Geometry: final body of the model. Coordinates: model frame, mm. A direction names the side the tool comes from. Give positions to 0.01 mm unless a question says otherwise; leave off trailing zeros. Order: outer loops, then holes, each group sorted by start corner. A loop starts at its lowest first (then second) coordinate and runs counter-clockwise, first axis right, second up. Notation, with made-up numbers: (57.25, 58.5) -> (115.25, 58.5) arc R23 cw to (115.25, 91.5) -> close; hole circle Ø4 at (-7.5, 74). An arc over 180 degrees is marked (long way). One line per question, with ' | ' between items.
from build123d import *

# Parameters (mm, degrees)
SKETCH1_R           = 13.97
BOSS_EXTRUDE2_DEPTH = 6.0000007
CUT_EXTRUDE1_DEPTH  = 3.81
SKETCH3_R           = 31.75
CUT_EXTRUDE2_DEPTH  = 0.3
SKETCH5_R           = 25.019
SKETCH5_R_2         = 13.97
BOSS_EXTRUDE3_DEPTH = 6.35
CUT_EXTRUDE3_START  = -0.3
SKETCH6_R           = 50.8
SKETCH6_R_2         = 31.75
CUT_EXTRUDE3_DEPTH  = 0.3


with BuildPart() as part:
    # Sketch1 → Boss-Extrude2 (new body)
    with BuildSketch(Plane(origin=(0, 0, 0), x_dir=(1, 0, 0), z_dir=(0, 1, 0))):
        with BuildLine():
            Line((35.405449863, 6.5405), (38.565312338, 6.5405))
            ThreePointArc((38.565312338, 6.5405), (27.795594479, 27.522107178), (6.9215, 38.498757042))
            Line((6.9215, 38.498757042), (6.9215, 35.332942957))
            ThreePointArc((6.9215, 35.332942957), (0.19391896, 36.003977776), (-6.5405, 35.405449863))
            Line((-6.5405, 35.405449863), (-6.5405, 38.565312338))
            ThreePointArc((-6.5405, 38.565312338), (-27.522107178, 27.795594479), (-38.498757042, 6.9215))
            Line((-38.498757042, 6.9215), (-35.332942957, 6.9215))
            ThreePointArc((-35.332942957, 6.9215), (-36.003977776, 0.19391896), (-35.405449863, -6.5405))
            Line((-35.405449863, -6.5405), (-38.565312338, -6.5405))
            ThreePointArc((-38.565312338, -6.5405), (-27.795594479, -27.522107178), (-6.9215, -38.498757042))
            Line((-6.9215, -38.498757042), (-6.9215, -35.332942957))
            ThreePointArc((-6.9215, -35.332942957), (-0.19391896, -36.003977776), (6.5405, -35.405449863))
            Line((6.5405, -35.405449863), (6.5405, -38.565312338))
            ThreePointArc((6.5405, -38.565312338), (27.522107178, -27.795594479), (38.498757042, -6.9215))
            Line((38.498757042, -6.9215), (35.332942957, -6.9215))
            ThreePointArc((35.332942957, -6.9215), (36.003977776, -0.19391896), (35.405449863, 6.5405))
        make_face()
        with Locations(Location((0, 0, 0), (0, 0, 270))):
            Circle(SKETCH1_R, mode=Mode.SUBTRACT)
    extrude(amount=BOSS_EXTRUDE2_DEPTH)

    # Sketch2 → Cut-Extrude1 (cut)
    with BuildSketch(Plane.XZ):
        with BuildLine():
            Line((17.377665752, -10.033), (-0.286554615, -40.628327152))
            ThreePointArc((-0.286554615, -40.628327152), (-2.416432138, -40.557415308), (-4.539661745, -40.374924792))
            Line((-4.539661745, -40.374924792), (8.196212586, -18.315743371))
            ThreePointArc((8.196212586, -18.315743371), (-13.440862054, 14.899247741), (17.377665752, -10.033))
        make_face()
    extrude(amount=-CUT_EXTRUDE1_DEPTH, mode=Mode.SUBTRACT)

    # Sketch3 → Cut-Extrude2 (cut)
    with BuildSketch(Plane.XZ):
        Circle(SKETCH3_R)
    extrude(amount=-CUT_EXTRUDE2_DEPTH, mode=Mode.SUBTRACT)

    # Sketch5 → Boss-Extrude3 (add)
    with BuildSketch(Plane(origin=(0, 6.0000007, 0), x_dir=(1, 0, 0), z_dir=(0, 1, 0))):
        with Locations(Location((0, 0, 0), (0, 0, 270))):
            Circle(SKETCH5_R)
        with Locations(Location((0, 0, 0), (0, 0, 270))):
            Circle(SKETCH5_R_2, mode=Mode.SUBTRACT)
    extrude(amount=BOSS_EXTRUDE3_DEPTH)

    # Sketch6 → Cut-Extrude3 (cut)
    with BuildSketch(Plane(origin=(0, 6.0000007, 0), x_dir=(1, 0, 0), z_dir=(0, 1, 0)).offset(CUT_EXTRUDE3_START)):
        Circle(SKETCH6_R)
        with Locations(Location((0, 0, 0), (0, 0, 270))):
            Circle(SKETCH6_R_2, mode=Mode.SUBTRACT)
    extrude(amount=CUT_EXTRUDE3_DEPTH, mode=Mode.SUBTRACT)


solid = part.part
1) Pull-direction query (X, two-part tool) for faces 4 (the flat face through (-6.922, 3, 37)), 5 (the cylindrical face through (27.283, 2.81, 28.031)), 6 (the flat face through (-32, 5.7, -6)); classes: +X half, -X half, draft (parallel to the pull), parting line (faces both ways), or undercut.
Check result:
face 4: undercut | face 5: +X half | face 6: draft
2) Section B-B on x = -4. Return loops of the section in (y, z).
Check result:
outline: (0, -35.78) -> (5.7, -35.78) -> (5.7, -31.5) -> (6, -31.5) -> (6, -24.7) -> (12.35, -24.7) -> (12.35, -13.39) -> (3.81, -13.39) -> (3.81, -19.66) -> (0.3, -19.66) -> (0.3, -31.5) -> (0, -31.5) -> close; (0, 31.5) -> (0.3, 31.5) -> (0.3, 19.66) -> (3.81, 19.66) -> (3.81, 13.39) -> (12.35, 13.39) -> (12.35, 24.7) -> (6, 24.7) -> (6, 31.5) -> (5.7, 31.5) -> (5.7, 35.78) -> (0, 35.78) -> close
3) Material intervals for probe 1 along X at (y, z) = (9, 0); probe 2 along Y at (x, z) = (-14.5, 17); probe 3 along X at (y, z) = (1.75, 0), sorted ascending. Write a range as from..to.
Check result:
probe 1: x = -25.02..-13.97, 13.97..25.02 | probe 2: y = 0.3..12.35 | probe 3: x = -36..-20.07, 20.07..36
4) Section A-A on z = 0. Return loops of the section in (x, y).
Check result:
outline: (-36, 0) -> (-31.75, 0) -> (-31.75, 0.3) -> (-20.07, 0.3) -> (-20.07, 3.81) -> (-13.97, 3.81) -> (-13.97, 12.35) -> (-25.02, 12.35) -> (-25.02, 6) -> (-31.75, 6) -> (-31.75, 5.7) -> (-36, 5.7) -> close; (13.97, 3.81) -> (20.07, 3.81) -> (20.07, 0.3) -> (31.75, 0.3) -> (31.75, 0) -> (36, 0) -> (36, 5.7) -> (31.75, 5.7) -> (31.75, 6) -> (25.02, 6) -> (25.02, 12.35) -> (13.97, 12.35) -> close
5) Section D-D on y = 10. Return loops of the section in (x, z).
Check result:
outline: circle Ø50.04 at (0, 0); hole circle Ø27.94 at (0, 0)
6) Set-up query: faces 1 (the flat face through (-6.54, 3, -37)), 2 (the flat face through (23.4, 6, -9.6)), 3 (the flat face through (10.009, 1.878, -22.796)). Return all of +Z, -Z, +X, -X, +Y, -Y with unobstructed straight access to the full face (end or side cutting, diameter ignored); none if empty.
Check result:
face 1: -Z, +Y, -Y | face 2: +Y | face 3: -Y
7) Contact query for flat-ended pins moving along their axis: pin 1 Ø2.5 at (y, z) = (1.5, -36.5) entering from +X; pin 2 Ø0.9 at (y, z) = (2.5, 36) entering from +X; pin 3 Ø12 at (x, z) = (-1, -8) entering from -Y. Output: stop coordinate, or through.
Check result:
pin 1: stops at x = 16.96 | pin 2: stops at x = 16.32 | pin 3: stops at y = 3.81
8) Section C-C on x = 21. Return loops of the section in (y, z), plus the area to 3 significant figures.
Check result:
outline: (0, -33) -> (5.7, -33) -> (5.7, -23.81) -> (6, -23.81) -> (6, -13.6) -> (12.35, -13.6) -> (12.35, 13.6) -> (6, 13.6) -> (6, 23.81) -> (5.7, 23.81) -> (5.7, 33) -> (0, 33) -> (0, 23.81) -> (0.3, 23.81) -> (0.3, -23.81) -> (0, -23.81) -> close | area: 549 mm^2
